Autodesk Fusion 360 part; units mm, degrees
sketch "Sketch1" plane through (0, 0, 0) normal (0, 0, 1) x (1, 0, 0)
  line L0 (50, -25) -> (-50, -25)
  line L1 (-50, -25) -> (-50, 25)
  line L2 (-50, 25) -> (50, 25)
  line L3 (50, 25) -> (50, -25)
  line L4 (50, -25) -> (-50, 25) construction
  line L5 (-50, -25) -> (50, 25) construction
  dimension "d1" = 100
  dimension "d2" = 50
extrude "Extrude1" add sketch "Sketch1" along normal blind 60
sketch "Sketch2" plane through (0, -25, 0) normal (0, -1, 0) x (1, 0, 0)
  line L0 (-50, 0) -> (50, 0)
  line L1 (50, 0) -> (50, 60)
  line L2 (50, 60) -> (-50, 60)
  line L3 (-50, 60) -> (-50, 0)
  line L4 (-50, 35.014) -> (-45.6262, 35.014)
  circle A0 centre (-19.3951, 34.5262) radius 26.2357
  line L5 (-25.6715, 60) -> (-25.6715, 25.0092)
  line L6 (-25.6715, 25.0092) -> (35, 25.0092)
  line L7 (35, 25.0092) -> (35, 60)
  line L8 (35, 30.0471) -> (-25.6715, 30.0471)
  line L9 (35, 30.0471) -> (35, 35.0471)
  line L10 (35, 35.0471) -> (50, 35.0471)
  dimension "d25" = 5
extrude "Extrude2" cut sketch "Sketch2" against normal blind 100 contours L2 A0 L7 L8 L9
extrude "Extrude3" cut sketch "Sketch2" against normal blind 100 contours L2 A0 | L2 A0 L5 L8
extrude "Extrude4" cut sketch "Sketch2" against normal blind 17.5 contours A0 L5 L6 L8 | A0 L6 L7 L8
extrude "Extrude5" cut sketch "Sketch2" against normal blind 100 contours L2 L3 L4 A0
sketch "Sketch3" plane through (-50, 0, 0) normal (-1, 0, 0) x (0, -1, 0)
  line L0 (25, 35.014) -> (-25, 35.014)
  line L1 (-25, 35.014) -> (-25, 0)
  line L2 (-25, 0) -> (25, 0)
  line L3 (25, 0) -> (25, 35.014)
  line L4 (-25, 0) -> (-15, 0)
  line L5 (25, 0) -> (15, 0)
  line L6 (15, 0) -> (15, 15)
  line L7 (-15, 0) -> (-15, 15)
  line L8 (-7.4, 15) -> (-7.4, 30)
  line L9 (7.4, 15) -> (7.4, 30)
  line L10 (7.4, 30) -> (-7.4, 30)
  line L11 (-15, 15) -> (-7.4, 15)
  line L12 (15, 15) -> (7.4, 15)
  dimension "d21" = 7.6
  dimension "d22" = 7.6
extrude "Extrude6" cut sketch "Sketch3" against normal blind 100 contours L2 L6 L7 L8 L9 L10 L11 L12
extrude "Extrude7" cut sketch "Sketch2" against normal blind 2 contours L1 L2 L7 L10
sketch "Sketch4" plane through (50, 0, 0) normal (1, 0, 0) x (0, 1, 0)
  line L0 (-23, 35.0471) -> (-25, 35.0471)
  line L1 (-25, 35.0471) -> (-25, 0)
  line L2 (-25, 0) -> (-15, 0)
  line L3 (-15, 0) -> (-15, 15)
  line L4 (-15, 15) -> (-7.4, 15)
  line L5 (-7.4, 15) -> (-7.4, 30)
  line L6 (-7.4, 30) -> (7.4, 30)
  line L7 (7.4, 30) -> (7.4, 15)
  line L8 (7.4, 15) -> (15, 15)
  line L9 (15, 15) -> (15, 0)
  line L10 (15, 0) -> (25, 0)
  line L11 (25, 0) -> (25, 60)
  line L12 (25, 60) -> (-23, 60)
  line L13 (-23, 60) -> (-23, 35.0471)
  line L14 (-25, 35.0471) -> (25, 35.0471)
  circle A0 centre (0, 35.0471) radius 12.5
  dimension "d28" = 25
extrude "Extrude8" cut sketch "Sketch4" against normal blind 50 contours L11 L12 L13 L14 A0
sketch "Sketch5" plane through (0, 25, 0) normal (0, 1, 0) x (-1, 0, 0)
  line L0 (-35, 35.0471) -> (-50, 35.0471)
  line L1 (-50, 35.0471) -> (-50, 0)
  line L2 (-50, 0) -> (50, 0)
  line L3 (50, 0) -> (50, 35.014)
  line L4 (50, 35.014) -> (45.6262, 35.014)
  arc A0 (45.6262, 35.014) -> (25.6715, 60) centre (19.3951, 34.5262) ccw
  line L5 (25.6715, 60) -> (25.6715, 30.0471)
  line L6 (25.6715, 30.0471) -> (-35, 30.0471)
  line L7 (-35, 30.0471) -> (-35, 35.0471)
  line L8 (25.6715, 30.0471) -> (25.6715, 25.0471)
  line L9 (25.6715, 25.0471) -> (-29.3285, 25.0471)
  line L10 (-29.3285, 25.0471) -> (-35, 30.0471)
  line L11 (-35, 30.0471) -> (-35, 17)
  line L12 (-29.3285, 25.0471) -> (-40, 25.0471)
  dimension "d31" = 5
  dimension "d32" = 55
extrude "Extrude9" cut sketch "Sketch5" against normal blind 17.5 contours L6 L8 L9 L10
extrude "Extrude10" cut sketch "Sketch5" against normal blind 17.5 contours L10 L11 L12
Here's how the part is built. I have some questions about the finished solid (model axes, mm). A direction names the side the tool comes from. Give positions to 0.01 mm unless a question says otherwise; leave off trailing zeros. Write each loop counter-clockwise with the first axis right and the second up, starting at its lowest first coordinate (ties: lowest second). Pieces come first, ordered by that corner, then holes.
(1) Imagine slicing it at A-A, the plane z = 17. Write out the boundary of the cut face in (x, y).
Output values:
outline: (-50, -25) - (50, -25) - (50, -7.4) - (-50, -7.4) - close; (-50, 7.4) - (50, 7.4) - (50, 25) - (-50, 25) - close
(2) On a 3-axis mill with a long thin cutter (end or side, diameter ignored), from which of +Z, -Z, +X, -X, +Y, -Y can I reach the whole of each face in a straight line? I mean faces 4 (the face through (-48, 0, 35.014)), 5 (the face through (-1, 15, 7)), 6 (the face through (42.605, 0.275, 47.544)), 7 (the face through (43, 19, 35.047)), 8 (the face through (42, -19, 35.047)). Say none if no direction works.
Output values:
face 4: +Z, -X, +Y, -Y
face 5: -Z, +X, -X
face 6: +Z, +X
face 7: +Z, +X, +Y
face 8: +Z, +X, -Y
(3) Will these pins go through, and if not, where does the flat tip stop? pin 1 (4 mm diameter, centred on x = 42.5, y = -18, fed in from +Z); pin 2 (2.5 mm diameter, centred on x = 2, y = -11, fed in from -Z); pin 3 (8 mm diameter, centred on y = 8.5, z = 11.5, fed in from +X); pin 4 (6 mm diameter, centred on x = 6.5, y = 14, fed in from +Z).
Output values:
pin 1: stops at z = 35.05
pin 2: stops at z = 15
pin 3: stops at x = 50
pin 4: stops at z = 25.05
(4) Imagine slicing it at C-C, the plane x = 3. Write out the boundary of the cut face in (y, z), and give its area (3 significant figures).
Output values:
outline: (-25, 0) - (-15, 0) - (-15, 15) - (-7.4, 15) - (-7.4, 30) - (7.4, 30) - (7.4, 15) - (15, 15) - (15, 0) - (25, 0) - (25, 25.05) - (7.5, 25.05) - (7.5, 30.05) - (-7.5, 30.05) - (-7.5, 25.01) - (-25, 25.01) - close
area: 655 mm2
(5) Imagine slicing it at B-B, the plane y = 0. Write out the boundary of the cut face in (x, z), and give its area (3 significant figures).
Output values:
outline: (-50, 30) - (50, 30) - (50, 47.55) - (35, 47.55) - (35, 30.05) - (-25.67, 30.05) - (-25.67, 60) arc R26.24 ccw to (-45.63, 35.01) - (-50, 35.01) - close
area: 756 mm2
(6) Imagine slicing it at D-D, the plane z = 41. Write out the boundary of the cut face in (x, y), and give its area (3 significant figures).
Output values:
outline: (-44.82, -25) - (-25.67, -25) - (-25.67, 25) - (-44.82, 25) - close; (35, -10.99) - (50, -10.99) - (50, 10.99) - (35, 10.99) - close
area: 1,290 mm2
(7) If I drill on L1, parallel to Y at x = -8, z = 17.5; L2, parallel to Y at x = -39, z = 13.5; L3, parallel to X at y = 11.5, z = 28, over which ranges is the centre line in solid material (lowest first)?
Output values:
L1: y = -25 to -7.4, 7.4 to 25
L2: y = -25 to -15, 15 to 25
L3: x = -50 to -25.67, 35 to 50
(8) Thinking about a two-plate mould opening in X: for faces 1 (the face through (-39.74, -0.35, 51.09)), 2 (the face through (-25.672, 0, 43)), 3 (the face through (-10, -25, 16)), which applies, pulls with the +X half, pulls with the -X half, needs draft (parallel to the pull), parting line crosses it, or undercut?
Output values:
face 1: pulls with the -X half
face 2: undercut
face 3: needs draft
